Can you work these out from the model? Positions are in its coordinate system, mm. Give positions to 0.01 mm unless a question says otherwise; leave off trailing zeros. Loops run counter-clockwise (first coordinate to the right, second up) from the corner with the lowest first, then second, coordinate; pieces in that order, holes last. Notation, with made-up numbers: (54, 65.25) - (101, 65.25) arc R5 cw to (101, 72.25) - close; hole circle Ø5 at (46.25, 76). An arc over 180 degrees is marked (long way). Answer as a JSON object with one key per item and string values. Group by question number.
Item 1: Suppose I cut it at D-D on z = 40.5. Write out the boundary of the cut face in (x, y).
Item 2: Suppose I cut it at A-A on z = 0. Write out the boundary of the cut face in (x, y) (3 decimals).
Item 3: Suppose I cut it at C-C on x = 1.35. Count the separate pieces of the cut face and the enclosed holes in it, and give its area (3 significant figures).
Item 4: Thinking about a two-plate mould opening in Y: for faces 1 (the cylindrical face through (0.986, 16.671, -52.937)), 2 (the cylindrical face through (0.986, -47.526, -0.391)), 3 (the flat face through (2, -41, -12)), which applies, pulls with the +Y half, pulls with the -Y half, needs draft (parallel to the pull), parting line crosses it, or undercut?
Item 5: Will these pins go through, and if not, where does the flat tip stop? pin 1 (1 mm diameter, centred on x = 1, z = 13, fed in from -Y); pin 2 (1.5 mm diameter, centred on y = -37.5, z = 18.5, fed in from +X).
Item 6: Please list where these lines run through material, in increasing order: L1, parallel to Z at x = 0.8, y = -33; L2, parallel to Z at x = 1.05, y = -35; L3, parallel to Y at x = 0.7, z = 36.
from build123d import *

# Parameters (mm, degrees)
SKETCH1_R           = 55.5
SKETCH1_R_2         = 42.495
BOSS_EXTRUDE1_DEPTH = 2
SKETCH2_R           = 3
CUT_EXTRUDE1_DEPTH  = 15


with BuildPart() as part:
    # Sketch1 → Boss-Extrude1 (new body)
    with BuildSketch(Plane(origin=(0, 0, 0), x_dir=(0, 0, -1), z_dir=(1, 0, 0))):
        Circle(SKETCH1_R)
        Circle(SKETCH1_R_2, mode=Mode.SUBTRACT)
    extrude(amount=BOSS_EXTRUDE1_DEPTH)

    # Sketch2 → Cut-Extrude1 (cut)
    with BuildSketch(Plane.ZY):
        with Locations((0, 50.5)):
            Circle(SKETCH2_R)
        with Locations((35.70889245, 35.70889245)):
            Circle(SKETCH2_R)
        with Locations((50.5, 0)):
            Circle(SKETCH2_R)
        with Locations((35.70889245, -35.70889245)):
            Circle(SKETCH2_R)
        with Locations((0, -50.5)):
            Circle(SKETCH2_R)
        with Locations((-35.70889245, -35.70889245)):
            Circle(SKETCH2_R)
        with Locations((-50.5, 0)):
            Circle(SKETCH2_R)
        with Locations((-35.70889245, 35.70889245)):
            Circle(SKETCH2_R)
    extrude(amount=-CUT_EXTRUDE1_DEPTH, mode=Mode.SUBTRACT)


solid = part.part
Worked out:
{
 "1": {"outline": "(0, -37.95) - (2, -37.95) - (2, -12.87) - (0, -12.87) - close; (0, 12.87) - (2, 12.87) - (2, 37.95) - (0, 37.95) - close"},
 "2": {"outline": "(0, -55.5) - (2, -55.5) - (2, -53.5) - (0, -53.5) - close; (0, -47.5) - (2, -47.5) - (2, -42.495) - (0, -42.495) - close; (0, 42.495) - (2, 42.495) - (2, 47.5) - (0, 47.5) - close; (0, 53.5) - (2, 53.5) - (2, 55.5) - (0, 55.5) - close"},
 "3": {"separate pieces": "1", "enclosed holes": "9", "area": "3,780 mm2"},
 "4": {"face 1": "parting line crosses it", "face 2": "undercut", "face 3": "needs draft"},
 "5": {"pin 1": "stops at y = -54.07", "pin 2": "stops at x = 2"},
 "6": {"L1": "z = -44.62 to -37, -34.42 to -26.77, 26.77 to 34.42, 37 to 44.62", "L2": "z = -43.07 to -38.62, -32.79 to -24.1, 24.1 to 32.79, 38.62 to 43.07", "L3": "y = -42.24 to -38.69, -32.72 to -22.58, 22.58 to 32.72, 38.69 to 42.24"}
}
